Model file for the job. Use its own axes, mm. Round coordinates to 2 decimals unless told otherwise and drop trailing zeros. Loops run counter-clockwise (first coordinate to the right, second up) from the corner with the lowest first, then second, coordinate; pieces in that order, holes last. Notation, with made-up numbers: M 11,34.5 L 68,34.5 A17 cw 68,38.5 Z; hole C -36,9 d2. An arc over 180 degrees is marked long. Use a Markdown table: item, result. Add a question column.
Item 1: Wall check: L1, parallel to X at y = 2.7, z = 44; L2, parallel to X at y = 1.95, z = 47.5; L3, parallel to X at y = 0.95, z = 74.5. Give the ranges that are in metal, low to high. Write a range as from..to.
Item 2: Pin check, flat tips, straight feed: P1, Ø7, axis at x = -3.72, z = 22.28, coming from the +Y side; P2, Ø6.5, axis at x = -3.72, z = 46.28, coming from the -Y side; P3, Ø2, axis at y = 2, z = 12, coming from the +X side; P4, Ø2, axis at x = 33, y = 2, coming from the -Z side. Stop position of each tip, or through.
Item 3: Saw through at C-C on y = 2.45. Give the number of separate pieces and of enclosed holes in the cut face, then the cut area to 3 significant figures.
Item 4: Saw through at A-A on x = -71. Write the cut outline in (y, z).
Item 5: Saw through at B-B on z = 54.5. Write the cut outline in (x, y).
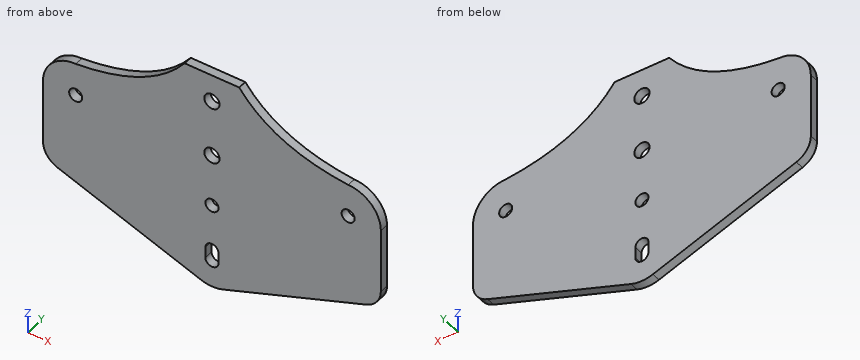
```python
from build123d import *

# Parameters (mm, degrees)
SKETCH2_R              = 3
SKETCH2_R_2            = 3.5
MAINPLATEEXTRUDE_DEPTH = 4


with BuildPart() as part:
    # Sketch2 → MainPlateExtrude (new body)
    with BuildSketch(Plane(origin=(0, 0, 0), x_dir=(1, 0, 0), z_dir=(0, 1, 0))):
        with BuildLine():
            Line((-81.215970545, -46.28367362), (-81.215970545, -16.925572983))
            ThreePointArc((-81.215970545, -16.925572983), (-79.384065752, -11.156498475), (-74.559526408, -7.501103014))
            Line((-74.559526408, -7.501103014), (-8.731304339, 15.853031333))
            ThreePointArc((-8.731304339, 15.853031333), (-3.715970545, 16.71632638), (1.299363248, 15.853031333))
            Line((1.299363248, 15.853031333), (67.127585317, -7.501103014))
            ThreePointArc((67.127585317, -7.501103014), (71.952124662, -11.156498475), (73.784029455, -16.925572983))
            Line((73.784029455, -16.925572983), (73.784029455, -46.28367362))
            ThreePointArc((73.784029455, -46.28367362), (69.390631173, -56.890275338), (58.784029455, -61.28367362))
            add(Edge.make_bspline(
                [(58.784029455, -61.28367362), (24.556467528, -64.469839896), (8.784029455, -84.862635588)],
                knots=[0, 0, 0, 0.615675344, 0.615675344, 0.615675344], degree=2))
            Line((8.784029455, -84.862635588), (-16.215970545, -84.862635588))
            add(Edge.make_bspline(
                [(-66.215970545, -61.28367362), (-31.988408619, -64.469839896), (-16.215970545, -84.862635588)],
                knots=[0, 0, 0, 0.615675344, 0.615675344, 0.615675344], degree=2))
            ThreePointArc((-66.215970545, -61.28367362), (-76.822572263, -56.890275338), (-81.215970545, -46.28367362))
        make_face()
        with Locations(Location((-66.215970545, -46.28367362, 0), (0, 0, 270))):
            Circle(SKETCH2_R, mode=Mode.SUBTRACT)
        with Locations(Location((58.784029455, -46.28367362, 0), (0, 0, 270))):
            Circle(SKETCH2_R, mode=Mode.SUBTRACT)
        with Locations(Location((-3.715970545, -46.28367362, 0), (0, 0, 270))):
            Circle(SKETCH2_R_2, mode=Mode.SUBTRACT)
        with Locations(Location((-3.715970545, -72.362635588, 0), (0, 0, 270))):
            Circle(SKETCH2_R_2, mode=Mode.SUBTRACT)
        with Locations(Location((-3.715970545, -22.28367362, 0), (0, 0, 270))):
            Circle(SKETCH2_R, mode=Mode.SUBTRACT)
        with BuildLine():
            Line((-0.715970545, 4.21632638), (-0.715970545, -0.78367362))
            ThreePointArc((-0.715970545, -0.78367362), (-3.715970545, -3.78367362), (-6.715970545, -0.78367362))
            Line((-6.715970545, -0.78367362), (-6.715970545, 4.21632638))
            ThreePointArc((-6.715970545, 4.21632638), (-3.715970545, 7.21632638), (-0.715970545, 4.21632638))
        make_face(mode=Mode.SUBTRACT)
    extrude(amount=MAINPLATEEXTRUDE_DEPTH)


solid = part.part
```
Entries:
| question | item | result |
|---|---|---|
| 1 | L1 | -81.22..-68.16, -64.27..-6.37, -1.06..56.84, 60.73..73.78 |
| 1 | L2 | -81.17..-68.96, -63.47..-7, -0.43..56.04, 61.53..73.73 |
| 1 | L3 | -26.89..-6.49, -0.94..19.46 |
| 2 | P1 | y = 4 |
| 2 | P2 | through |
| 2 | P3 | x = 72.98 |
| 2 | P4 | z = -4.96 |
| 3 | separate pieces | 1 |
| 3 | enclosed holes | 6 |
| 3 | area | 11,100 mm2 |
| 4 | outline | M 0,6.24 L 4,6.24 L 4,60.5 L 0,60.5 Z |
| 5 | outline | M -78.77,0 L 71.33,0 L 71.33,4 L -78.77,4 Z |
